Check sheet for the modelled part. Datum: model origin and axes. Units: mm. Face numbers are marked on the shaded views. A direction names the side the tool comes from. Round coordinates to 2 decimals unless told otherwise and drop trailing zeros. Order: outer loops, then holes, each group sorted by start corner. A loop starts at its lowest first (then second) coordinate and runs counter-clockwise, first axis right, second up.
Q1. Cross-section at C-C on z = 7.25. Record the cut outline in (x, y).
Q2. Set-up check for the marked faces 1 and 2: record each of +Z, -Z, +X, -X, +Y, -Y from which the full face is reachable in a straight line by a thin tool's end or side.
Q3. Cross-section at B-B on y = 0. Record the cut outline in (x, z), then the cut area to 3 significant figures.
Q4. Cross-section at A-A on z = 0. Record the cut outline in (x, y).
Q5. Mould release check, pull along Y, two halves, no side actions. Record for the marked faces 3, 4 and 5: +Y half, -Y half, draft (parallel to the pull), parting line (faces both ways), or undercut.
Q6. Scan lines: probe 1 along Y at (x, z) = (10.1, 0); probe 2 along X at (y, z) = (-5.25, 1.25); probe 3 along Z at (x, y) = (1.25, -7.25). Record each from-to range of solid material in increasing order.
Q7. Depth check by flat-ended pin: P1, Ø8, axis at x = -1, z = -2.5, coming from the +Y side. Enter the tip coordinate at first touch or a pass-through.
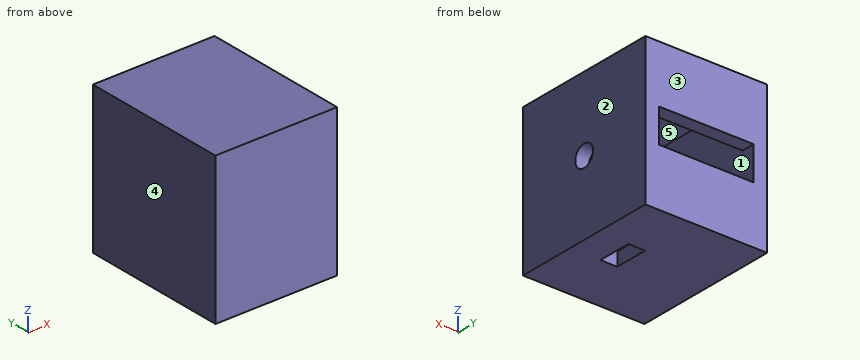
from build123d import *

# Parameters (mm, degrees)
SKETCH2_W           = 22.987
SKETCH2_H           = 27.94
SKETCH2_W_2         = 17.907
SKETCH2_H_2         = 22.86
BOSS_EXTRUDE1_DEPTH = 13.97
SKETCH3_W           = 17.907
SKETCH3_H           = 22.86
BOSS_EXTRUDE2_DEPTH = 2.54
SKETCH4_W           = 17.907
SKETCH4_H           = 8.255
BOSS_EXTRUDE3_DEPTH = 2.54
SKETCH6_R           = 2.032
CUT_EXTRUDE2_DEPTH  = 2.54
SKETCH7_W           = 3.175
SKETCH7_H           = 6.35
CUT_EXTRUDE3_DEPTH  = 2.54


with BuildPart() as part:
    # Sketch2 → Boss-Extrude1 (new, symmetric)
    with BuildSketch(Plane(origin=(0, 0, 0), x_dir=(1, 0, 0), z_dir=(0, 1, 0))):
        Rectangle(SKETCH2_W, SKETCH2_H)
        Rectangle(SKETCH2_W_2, SKETCH2_H_2, mode=Mode.SUBTRACT)
    extrude(amount=BOSS_EXTRUDE1_DEPTH, both=True)

    # Sketch3 → Boss-Extrude2 (add)
    with BuildSketch(Plane.XZ.offset(13.97)):
        Rectangle(SKETCH3_W, SKETCH3_H)
    extrude(amount=-BOSS_EXTRUDE2_DEPTH)

    # Sketch4 → Boss-Extrude3 (add)
    with BuildSketch(Plane(origin=(0, 13.97, 0), x_dir=(1, 0, 0), z_dir=(0, 1, 0))):
        with Locations((0, 7.3025)):
            Rectangle(SKETCH4_W, SKETCH4_H)
        with Locations((0, -7.3025)):
            Rectangle(SKETCH4_W, SKETCH4_H)
    extrude(amount=-BOSS_EXTRUDE3_DEPTH)

    # Sketch6 → Cut-Extrude2 (cut)
    with BuildSketch(Plane(origin=(11.4935, 0, 0), x_dir=(0, 0, -1), z_dir=(1, 0, 0))):
        Circle(SKETCH6_R)
    extrude(amount=-CUT_EXTRUDE2_DEPTH, mode=Mode.SUBTRACT)

    # Sketch7 → Cut-Extrude3 (cut)
    with BuildSketch(Plane(origin=(0, 0, -13.97), x_dir=(-1, 0, 0), z_dir=(0, 0, -1))):
        with Locations((-4.191, 0)):
            Rectangle(SKETCH7_W, SKETCH7_H)
    extrude(amount=-CUT_EXTRUDE3_DEPTH, mode=Mode.SUBTRACT)


solid = part.part
Results found:
1. outline: (-11.49, -13.97) - (11.49, -13.97) - (11.49, 13.97) - (-11.49, 13.97) - close; hole (-8.95, -11.43) - (8.95, -11.43) - (8.95, 11.43) - (-8.95, 11.43) - close
2. face 1: none
2. face 2: +Z, -Z, +X, +Y, -Y
3. outline: (-11.49, -13.97) - (2.6, -13.97) - (2.6, -11.43) - (-8.95, -11.43) - (-8.95, 11.43) - (8.95, 11.43) - (8.95, 2.03) - (11.49, 2.03) - (11.49, 13.97) - (-11.49, 13.97) - close; (5.78, -13.97) - (11.49, -13.97) - (11.49, -2.03) - (8.95, -2.03) - (8.95, -11.43) - (5.78, -11.43) - close
3. area: 215 mm2
4. outline: (-11.49, -13.97) - (11.49, -13.97) - (11.49, -2.03) - (8.95, -2.03) - (8.95, -11.43) - (-8.95, -11.43) - (-8.95, 13.97) - (-11.49, 13.97) - close; (8.95, 2.03) - (11.49, 2.03) - (11.49, 13.97) - (8.95, 13.97) - close
5. face 3: +Y half
5. face 4: draft
5. face 5: undercut
6. probe 1: y = -13.97 to -2.03, 2.03 to 13.97
6. probe 2: x = -11.49 to -8.95, 8.95 to 11.49
6. probe 3: z = -13.97 to -11.43, 11.43 to 13.97
7. P1: stops at y = 13.97
